CAD build for the part. Positions are in the model's coordinates, mm. Face numbers are marked on the shaded views. Give positions to 0.01 mm unless a question says otherwise; leave off trailing zeros. Loops run counter-clockwise (first coordinate to the right, second up) from the corner with the lowest first, then second, coordinate; pieces in that order, holes last.
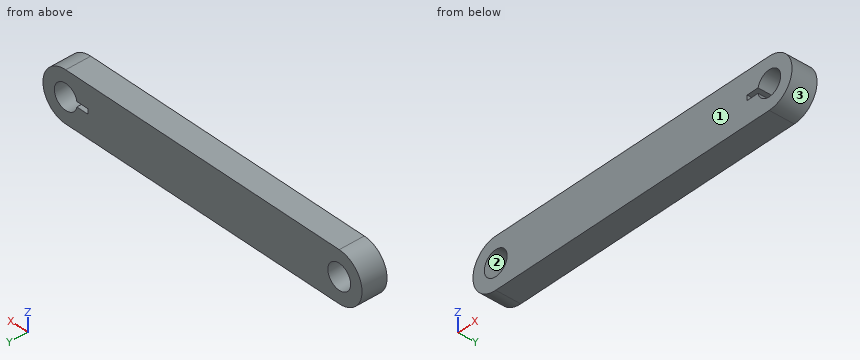
```python
from build123d import *

# Parameters (mm, degrees)
BOSS_EXTRUDE1_DEPTH = 6.35
CUT_EXTRUDE2_DEPTH  = 84.037024874
SKETCH4_R           = 3.175
CUT_EXTRUDE3_DEPTH  = 84.037024874


with BuildPart() as part:
    # Sketch1 → Boss-Extrude1 (new body)
    with BuildSketch(Plane(origin=(0, 0, 0), x_dir=(1, 0, 0), z_dir=(0, 1, 0))):
        with BuildLine():
            Line((0, -6.35), (-76.2, -6.35))
            ThreePointArc((-76.2, -6.35), (-82.55, 0), (-76.2, 6.35))
            Line((-76.2, 6.35), (0, 6.35))
            ThreePointArc((0, 6.35), (6.35, 0), (0, -6.35))
        make_face()
    extrude(amount=BOSS_EXTRUDE1_DEPTH)

    # Sketch3 → Cut-Extrude2 (cut, through all)
    with BuildSketch(Plane(origin=(0, 6.35, 0), x_dir=(1, 0, 0), z_dir=(0, 1, 0))):
        with BuildLine():
            Line((-3.110851973, 0.635), (-6.158851973, 0.635))
            Line((-6.158851973, 0.635), (-6.158851973, -0.635))
            Line((-6.158851973, -0.635), (-3.110851973, -0.635))
            ThreePointArc((-3.110851973, -0.635), (3.175, 0), (-3.110851973, 0.635))
        make_face()
    extrude(amount=-CUT_EXTRUDE2_DEPTH, mode=Mode.SUBTRACT)

    # Sketch4 → Cut-Extrude3 (cut, through all)
    with BuildSketch(Plane(origin=(0, 6.35, 0), x_dir=(1, 0, 0), z_dir=(0, 1, 0))):
        with Locations(Location((-76.2, 0, 0), (0, 0, 270))):
            Circle(SKETCH4_R)
    extrude(amount=-CUT_EXTRUDE3_DEPTH, mode=Mode.SUBTRACT)


solid = part.part
```
1. Probe line 1 along X through (y, z) = (3.25, 0) (3 decimals); line 2 along Z through (x, y) = (-5.5, 2.5) (3 decimals); line 3 along X through (y, z) = (5.5, 0.5). List the from-to ranges inside material, lowest first.
Responses:
line 1: x = -82.55 to -79.375, -73.025 to -6.159, 3.175 to 6.35
line 2: z = -6.35 to -0.635, 0.635 to 6.35
line 3: x = -82.53 to -79.34, -73.06 to -6.16, 3.14 to 6.33
2. Saw through at C-C, the plane z = 4. List the corners of the cut face in (x, y), and give its area (3 significant figures).
Responses:
outline: (-81.13, 0) - (4.93, 0) - (4.93, 6.35) - (-81.13, 6.35) - close
area: 547 mm2
3. Pull direction X, two halves, no side cores. Call the marked faces 1, 2 and 3: released by +X, released by -X, zero draft, split by the parting line, or undercut.
Responses:
face 1: zero draft
face 2: undercut
face 3: released by +X
4. Saw through at B-B, the plane z = -2. List the corners of the cut face in (x, y), and give its area (3 significant figures).
Responses:
outline: (-82.23, 0) - (-78.67, 0) - (-78.67, 6.35) - (-82.23, 6.35) - close; (-73.73, 0) - (-2.47, 0) - (-2.47, 6.35) - (-73.73, 6.35) - close; (2.47, 0) - (6.03, 0) - (6.03, 6.35) - (2.47, 6.35) - close
area: 498 mm2
5. Drop flat-ended pins along their axis: pin 1 (3 mm diameter, centred on y = 5.5, z = 3, fed in from -X); pin 2 (4 mm diameter, centred on x = -76.2, z = 0, fed in from -Y) (3 decimals). Give the stop position or say it passes through.
Responses:
pin 1: stops at x = -82.37
pin 2: passes through
6. Saw through at A-A, the plane y = 4.5. List the corners of the cut face in (x, z) (3 decimals), and give its area (3 significant figures).
Responses:
outline: (-76.2, -6.35) - (0, -6.35) arc R6.35 ccw to (0, 6.35) - (-76.2, 6.35) arc R6.35 ccw to start; hole circle Ø6.35 at (-76.2, 0); hole (-6.159, -0.635) - (-3.111, -0.635) arc R3.175 ccw (long way) to (-3.111, 0.635) - (-6.159, 0.635) - close
area: 1,030 mm2
